Could you check a few things on this model? Use its own coordinates, in mm. Face numbers are marked on the shaded views. Give positions to 0.01 mm unless a question says otherwise; leave off trailing zeros. Write each loop counter-clockwise with the first axis right and the second up, starting at its lowest first coordinate (ties: lowest second). Pieces come first, ordered by that corner, then holes. Notation, with made-up numbers: (-5.5, -23.5) - (13.5, -23.5) arc R37 ccw to (13.5, 15.5) - close; hole circle Ø4 at (67, 80). An arc over 180 degrees is marked (long way). Use one line per item in the form item = value.
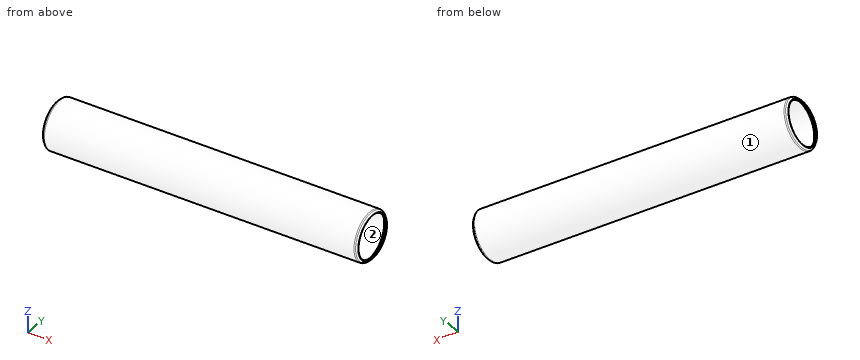
Autodesk Inventor part; units mm, degrees
ref_plane "cp1_XY" through (66.7449, 10.2553, 0) normal (1, 0, 0) x (0, 0, -1)
ref_plane "cp1_YZ" through (66.7449, 10.2553, 0) normal (0, 0, -1) x (0, 1, 0)
ref_plane "cp1_ZX" through (66.7449, 10.2553, 0) normal (0, 1, 0) x (1, 0, 0)
sketch "Sketch_1" plane through (0, 0, 0) normal (0, 0, 1) x (1, 0, 0)
  line L0 (133.4897, 0) -> (0, 0)
  arc A0 (-0.6395, 9.3472) -> (-0.6395, 9.1676) centre (-0.5497, 9.2574) ccw
  line L1 (-0.6395, 9.1676) -> (-0.381, 8.9091)
  line L2 (-0.381, 8.9091) -> (0, 8.9091)
  line L3 (0, 8.9091) -> (0.762, 9.671)
  line L4 (0.762, 9.671) -> (132.7277, 9.671)
  line L5 (132.7277, 9.671) -> (133.4897, 8.9091)
  line L6 (133.4897, 8.9091) -> (133.8707, 8.9091)
  line L7 (133.8707, 8.9091) -> (134.1292, 9.1676)
  arc A1 (134.1292, 9.1676) -> (134.1292, 9.3472) centre (134.0394, 9.2574) ccw
  line L8 (134.1292, 9.3472) -> (133.4443, 10.0321)
  arc A2 (133.4443, 10.0321) -> (132.9055, 10.2553) centre (132.9055, 9.4933) ccw
  line L9 (132.9055, 10.2553) -> (0.5842, 10.2553)
  arc A3 (0.5842, 10.2553) -> (0.0454, 10.0321) centre (0.5842, 9.4933) ccw
  line L10 (0.0454, 10.0321) -> (-0.6395, 9.3472)
revolve "Revolution1" add sketch "Sketch_1" angle 360 about axis through (133.4897, 0, 0) along (1, 0, 0)
ref_plane "cp1_XY" through (66.7449, 10.2553, 0) normal (1, 0, 0) x (0, 0, -1)
ref_plane "cp1_YZ" through (66.7449, 10.2553, 0) normal (0, 0, -1) x (0, 1, 0)
ref_plane "cp1_ZX" through (66.7449, 10.2553, 0) normal (0, 1, 0) x (1, 0, 0)
ref_plane "cp2_XY" through (66.7449, 0, -10.2553) normal (1, 0, 0) x (0, 0, -1)
ref_plane "cp2_YZ" through (66.7449, 0, -10.2553) normal (0, 0, -1) x (0, 1, 0)
ref_plane "cp2_ZX" through (66.7449, 0, -10.2553) normal (0, 1, 0) x (1, 0, 0)
ref_plane "cp3_XY" through (66.7449, -10.2553, 0) normal (1, 0, 0) x (0, 0, -1)
ref_plane "cp3_YZ" through (66.7449, -10.2553, 0) normal (0, 0, -1) x (0, 1, 0)
ref_plane "cp3_ZX" through (66.7449, -10.2553, 0) normal (0, 1, 0) x (1, 0, 0)
ref_plane "cp4_XY" through (66.7449, 0, 10.2553) normal (1, 0, 0) x (0, 0, -1)
ref_plane "cp4_YZ" through (66.7449, 0, 10.2553) normal (0, 0, -1) x (0, 1, 0)
ref_plane "cp4_ZX" through (66.7449, 0, 10.2553) normal (0, 1, 0) x (1, 0, 0)
ref_plane "tube_front_XY" through (0, 0, 0) normal (1, 0, 0) x (0, 0, -1)
ref_plane "tube_front_YZ" through (0, 0, 0) normal (0, 0, -1) x (0, 1, 0)
ref_plane "tube_front_ZX" through (0, 0, 0) normal (0, 1, 0) x (1, 0, 0)
ref_plane "tube_rear_XY" through (133.4897, 0, 0) normal (1, 0, 0) x (0, 0, -1)
ref_plane "tube_rear_YZ" through (133.4897, 0, 0) normal (0, 0, -1) x (0, 1, 0)
ref_plane "tube_rear_ZX" through (133.4897, 0, 0) normal (0, 1, 0) x (1, 0, 0)
properties part number "04R-5.25550C"
1. If I drill on line 1 (Z direction, x = -0.3, y = 0); line 2 (Z direction, x = 79.5, y = 0); line 3 (Y direction, x = 34, z = -5), over which ranges is the centre line in solid material (lowest first)? Write a range as from..to.
Response values:
line_1 = -9.69..-8.91, 8.91..9.69
line_2 = -10.26..-9.67, 9.67..10.26
line_3 = -8.95..-8.28, 8.28..8.95
2. For pin 1 (2 mm diameter, centred on x = 77, y = 2, fed in from +Z); pin 2 (6 mm diameter, centred on x = 90.5, y = 3.5, fed in from -Z); pin 3 (4 mm diameter, centred on x = 105, z = -6, fed in from -Y), each with a flat end and sliding along its axis, tell me the tip position at first contact or that it passes through.
Response values:
pin_1 = 10.21
pin_2 = -10.24
pin_3 = -9.44
3. Imagine slicing it at C-C, the plane x = 26. List the corners of the cut face in (y, z) for me.
Response values:
outline = circle Ø20.51 at (0, 0); hole circle Ø19.34 at (0, 0)
4. If we mould it in two halves opening along Z, with no side actions, what happens to the marked faces 1 and 2? For each: pulls with the +Z half, pulls with the -Z half, needs draft (parallel to the pull), parting line crosses it, or undercut.
Response values:
face_1 = parting line crosses it
face_2 = undercut
5. Imagine slicing it at A-A, the plane y = 0. List the corners of the cut face in (x, z) for me.
Response values:
outline = (-0.64, -9.35) - (0.05, -10.03) arc R0.76 ccw to (0.58, -10.26) - (132.91, -10.26) arc R0.76 ccw to (133.44, -10.03) - (134.13, -9.35) arc R0.13 ccw to (134.13, -9.17) - (133.87, -8.91) - (133.49, -8.91) - (132.73, -9.67) - (0.76, -9.67) - (0, -8.91) - (-0.38, -8.91) - (-0.64, -9.17) arc R0.13 ccw to start; (-0.64, 9.17) - (-0.38, 8.91) - (0, 8.91) - (0.76, 9.67) - (132.73, 9.67) - (133.49, 8.91) - (133.87, 8.91) - (134.13, 9.17) arc R0.13 ccw to (134.13, 9.35) - (133.44, 10.03) arc R0.76 ccw to (132.91, 10.26) - (0.58, 10.26) arc R0.76 ccw to (0.05, 10.03) - (-0.64, 9.35) arc R0.13 ccw to start
